Read the model definition and answer for the solid it produces. Units are mm, in the model's axes. A direction names the side the tool comes from. Coordinates: 2 decimals unless noted, no trailing zeros. Write each loop counter-clockwise with the first axis right and the second up, starting at its lowest first coordinate (ties: lowest second). Pieces come first, ordered by that corner, then holes. Notation, with made-up numbers: (70, 16) -> (109, 16) arc R9 ccw to (109, 33) -> close; hole circle Ø10 at (-13, -19.5). An arc over 180 degrees is marked (long way). Answer in a Markdown table with one row per item. Add a question column.
Item 1: Section A-A on y = -26.55 is taken. Write down the section's boundary in (x, z).
Item 2: Section B-B on z = 26 is taken. Write down the section's boundary in (x, y), then the cut area to 3 significant figures.
Item 3: Section D-D on x = -5.5 is taken. Write down the section's boundary in (y, z).
Item 4: Section C-C on x = 7 is taken. Write down the section's boundary in (y, z), then the cut area to 3 significant figures.
Item 5: Straight lines are drawn through the part: line 1 (Z direction, x = 3, y = -21); line 2 (Y direction, x = -1, z = 2); line 3 (X direction, y = -8, z = 27.5). For each, find the intervals that lie inside material, in ascending order. Write a range as from..to.
Item 6: Which of the six approach directions +Z, -Z, +X, -X, +Y, -Y give full straight-line access (tool end or side, diameter ignored) to faces 1 (the face through (7, -5.25, 15)), 2 (the face through (1, 5.25, 27)), 3 (the face through (3.5, 12.5, 15.2))?
Item 7: For a pull along Y with two mould halves and no side action, classify faces 4 (the face through (15.5, 0, 15)), 5 (the face through (-0.03, -47.2, 8.66)), 6 (the face through (7.43, -14.75, 15.21)) as +Y half, -Y half, draft (parallel to the pull), parting line (faces both ways), or undercut.
Item 8: Given pin 1 Ø8.5 at (y, z) = (-2.5, 10) entering from -X; pin 2 Ø15 at (y, z) = (-58.5, 19.5) entering from +X; pin 3 Ø3 at (y, z) = (-52.5, 15) entering from -X; pin 4 Ø3 at (y, z) = (-21.25, 15) entering from -X, each flat-ended and moving along its own axis, determine where each tip first touches the part or whether it passes through.
```python
from build123d import *

# Parameters (mm, degrees)
BOSS_EXTRUDE1_DEPTH = 30
CUT_EXTRUDE1_DEPTH  = 30
BOSS_EXTRUDE3_DEPTH = 30
SKETCH5_W           = 8
SKETCH5_H           = 30
BOSS_EXTRUDE4_DEPTH = 50
SKETCH6_R           = 1.65
CUT_EXTRUDE2_DEPTH  = 40
CUT_EXTRUDE3_DEPTH  = 65
FILLET1_R           = 5
FILLET3_R           = 1
FILLET4_R           = 1


with BuildPart() as part:
    # Sketch1 → Boss-Extrude1 (new body)
    with BuildSketch(Plane.XY):
        Polygon((-14.5, 13.25), (-14.5, 5.25), (15, 5.25), (15.5, 5.25), (15.5, -5.25), (15, -5.25), (-2, -5.25), (-2, -8.570490336), (-2, -29.25), (6, -29.25), (6, -13.25), (23, -13.25), (23, 13.25), align=None)
    extrude(amount=BOSS_EXTRUDE1_DEPTH)

    # Sketch3 → Cut-Extrude1 (cut)
    with BuildSketch(Plane.XY.offset(30)):
        Polygon((1.5, 13.25), (9.5, 13.25), (5.5, 11.75), align=None)
    extrude(amount=-CUT_EXTRUDE1_DEPTH, mode=Mode.SUBTRACT)

    # Sketch4 → Boss-Extrude3 (add)
    with BuildSketch(Plane.ZY.offset(14.5)):
        Polygon((5, 5.25), (25, 5.25), (15, 2.25), align=None)
    extrude(amount=-BOSS_EXTRUDE3_DEPTH)

    # Sketch5 → Boss-Extrude4 (add)
    with BuildSketch(Plane.XZ.offset(29.25)):
        with Locations((2, 15)):
            Rectangle(SKETCH5_W, SKETCH5_H)
    extrude(amount=BOSS_EXTRUDE4_DEPTH)

    # Sketch6 → Cut-Extrude2 (cut)
    with BuildSketch(Plane(origin=(6, 0, 0), x_dir=(0, 0, -1), z_dir=(1, 0, 0))):
        with BuildLine():
            ThreePointArc((-13.35, -31.85), (-13.833273811, -30.683273811), (-15, -30.2))
            Line((-15, -30.2), (-15, -33.5))
            ThreePointArc((-15, -33.5), (-13.833273811, -33.016726189), (-13.35, -31.85))
        make_face()
        with BuildLine():
            Line((-15, -33.5), (-15, -30.2))
            ThreePointArc((-15, -30.2), (-16.65, -31.85), (-15, -33.5))
        make_face()
        with BuildLine():
            ThreePointArc((-13.35, -37.15), (-13.833273811, -35.983273811), (-15, -35.5))
            Line((-15, -35.5), (-15, -38.8))
            ThreePointArc((-15, -38.8), (-13.833273811, -38.316726189), (-13.35, -37.15))
        make_face()
        with BuildLine():
            Line((-15, -38.8), (-15, -35.5))
            ThreePointArc((-15, -35.5), (-16.65, -37.15), (-15, -38.8))
        make_face()
        with BuildLine():
            ThreePointArc((-13.35, -42.45), (-13.833273811, -41.283273811), (-15, -40.8))
            Line((-15, -40.8), (-15, -44.1))
            ThreePointArc((-15, -44.1), (-13.833273811, -43.616726189), (-13.35, -42.45))
        make_face()
        with BuildLine():
            Line((-15, -44.1), (-15, -40.8))
            ThreePointArc((-15, -40.8), (-16.65, -42.45), (-15, -44.1))
        make_face()
        with BuildLine():
            ThreePointArc((-13.35, -47.75), (-13.833273811, -46.583273811), (-15, -46.1))
            Line((-15, -46.1), (-15, -49.4))
            ThreePointArc((-15, -49.4), (-13.833273811, -48.916726189), (-13.35, -47.75))
        make_face()
        with BuildLine():
            Line((-15, -49.4), (-15, -46.1))
            ThreePointArc((-15, -46.1), (-16.65, -47.75), (-15, -49.4))
        make_face()
        with BuildLine():
            ThreePointArc((-13.35, -53.05), (-13.833273811, -51.883273811), (-15, -51.4))
            Line((-15, -51.4), (-15, -54.7))
            ThreePointArc((-15, -54.7), (-13.833273811, -54.216726189), (-13.35, -53.05))
        make_face()
        with BuildLine():
            Line((-15, -54.7), (-15, -51.4))
            ThreePointArc((-15, -51.4), (-16.65, -53.05), (-15, -54.7))
        make_face()
        with BuildLine():
            ThreePointArc((-13.35, -58.35), (-13.833273811, -57.183273811), (-15, -56.7))
            Line((-15, -56.7), (-15, -60))
            ThreePointArc((-15, -60), (-13.833273811, -59.516726189), (-13.35, -58.35))
        make_face()
        with BuildLine():
            Line((-15, -60), (-15, -56.7))
            ThreePointArc((-15, -56.7), (-16.65, -58.35), (-15, -60))
        make_face()
        with BuildLine():
            ThreePointArc((-13.35, -63.65), (-13.833273811, -62.483273811), (-15, -62))
            Line((-15, -62), (-15, -65.3))
            ThreePointArc((-15, -65.3), (-13.833273811, -64.816726189), (-13.35, -63.65))
        make_face()
        with BuildLine():
            Line((-15, -65.3), (-15, -62))
            ThreePointArc((-15, -62), (-16.65, -63.65), (-15, -65.3))
        make_face()
        with BuildLine():
            ThreePointArc((-13.35, -68.95), (-13.833273811, -67.783273811), (-15, -67.3))
            Line((-15, -67.3), (-15, -70.6))
            ThreePointArc((-15, -70.6), (-13.833273811, -70.116726189), (-13.35, -68.95))
        make_face()
        with BuildLine():
            Line((-15, -70.6), (-15, -67.3))
            ThreePointArc((-15, -67.3), (-16.65, -68.95), (-15, -70.6))
        make_face()
        with BuildLine():
            ThreePointArc((-13.35, -74.25), (-13.833273811, -73.083273811), (-15, -72.6))
            Line((-15, -72.6), (-15, -75.9))
            ThreePointArc((-15, -75.9), (-13.833273811, -75.416726189), (-13.35, -74.25))
        make_face()
        with BuildLine():
            Line((-15, -75.9), (-15, -72.6))
            ThreePointArc((-15, -72.6), (-16.65, -74.25), (-15, -75.9))
        make_face()
        with Locations(Location((-15, -26.55, 0), (0, 0, 90))):
            Circle(SKETCH6_R)
        with Locations(Location((-15, -21.25, 0), (0, 0, 90))):
            Circle(SKETCH6_R)
    extrude(amount=-CUT_EXTRUDE2_DEPTH, mode=Mode.SUBTRACT)

    # Sketch7 → Cut-Extrude3 (cut)
    with BuildSketch(Plane.XZ.offset(79.25)):
        Polygon((-2, 27.5), (-2, 2.5), (2, 15), align=None)
    extrude(amount=-CUT_EXTRUDE3_DEPTH, mode=Mode.SUBTRACT)

    # Fillet1
    fillet1_edges = [part.edges().sort_by_distance(p)[0] for p in [
        (23, 13.25, 15),
        (23, -13.25, 15),
        (6, -13.25, 15),
    ]]
    fillet(fillet1_edges, radius=FILLET1_R)

    # Fillet3
    fillet3_edges = [part.edges().sort_by_distance(p)[0] for p in [
        (6, -79.25, 15),
    ]]
    fillet(fillet3_edges, radius=FILLET3_R)

    # Fillet4
    fillet4_edges = [part.edges().sort_by_distance(p)[0] for p in [
        (-14.5, 5.25, 27.5),
        (-14.5, 13.25, 15),
        (-14.5, 5.25, 2.5),
        (-14.5, 3.75, 20),
        (-14.5, 3.75, 10),
    ]]
    fillet(fillet4_edges, radius=FILLET4_R)


solid = part.part
```
Results below:
| question | item | result |
|---|---|---|
| 1 | outline | (-2, 0) -> (6, 0) -> (6, 13.35) -> (1.47, 13.35) -> (-2, 2.5) -> close; (-2, 27.5) -> (1.47, 16.65) -> (6, 16.65) -> (6, 30) -> (-2, 30) -> close |
| 2 | outline | (-14.5, 6.25) arc R1 ccw to (-13.5, 5.25) -> (15.5, 5.25) -> (15.5, -5.25) -> (-2, -5.25) -> (-2, -14.25) -> (-1.52, -14.25) -> (-1.52, -79.25) -> (5, -79.25) arc R1 ccw to (6, -78.25) -> (6, -18.25) arc R5 cw to (11, -13.25) -> (18, -13.25) arc R5 ccw to (23, -8.25) -> (23, 8.25) arc R5 ccw to (18, 13.25) -> (9.5, 13.25) -> (5.5, 11.75) -> (1.5, 13.25) -> (-13.5, 13.25) arc R1 ccw to (-14.5, 12.25) -> close |
| 2 | area | 1,060 mm2 |
| 3 | outline | (2.25, 15) -> (5.25, 5) -> (5.25, 0) -> (13.25, 0) -> (13.25, 30) -> (5.25, 30) -> (5.25, 25) -> close |
| 4 | outline | (-15.25, 0) -> (-5.25, 0) -> (-5.25, 30) -> (-15.25, 30) -> close; (2.25, 15) -> (5.25, 5) -> (5.25, 0) -> (12.31, 0) -> (12.31, 30) -> (5.25, 30) -> (5.25, 25) -> close |
| 4 | area | 542 mm2 |
| 5 | line 1 | z = 0..13.37, 16.63..30 |
| 5 | line 2 | y = -79.25..-5.25, 5.25..13.25 |
| 5 | line 3 | x = -2..23 |
| 6 | face 1 | +Z, -Z, -X |
| 6 | face 2 | +Z, -X |
| 6 | face 3 | +Z, -Z, +Y |
| 7 | face 4 | undercut |
| 7 | face 5 | draft |
| 7 | face 6 | -Y half |
| 8 | pin 1 | stops at x = -2 |
| 8 | pin 2 | stops at x = 6 |
| 8 | pin 3 | stops at x = 1.52 |
| 8 | pin 4 | passes through |
